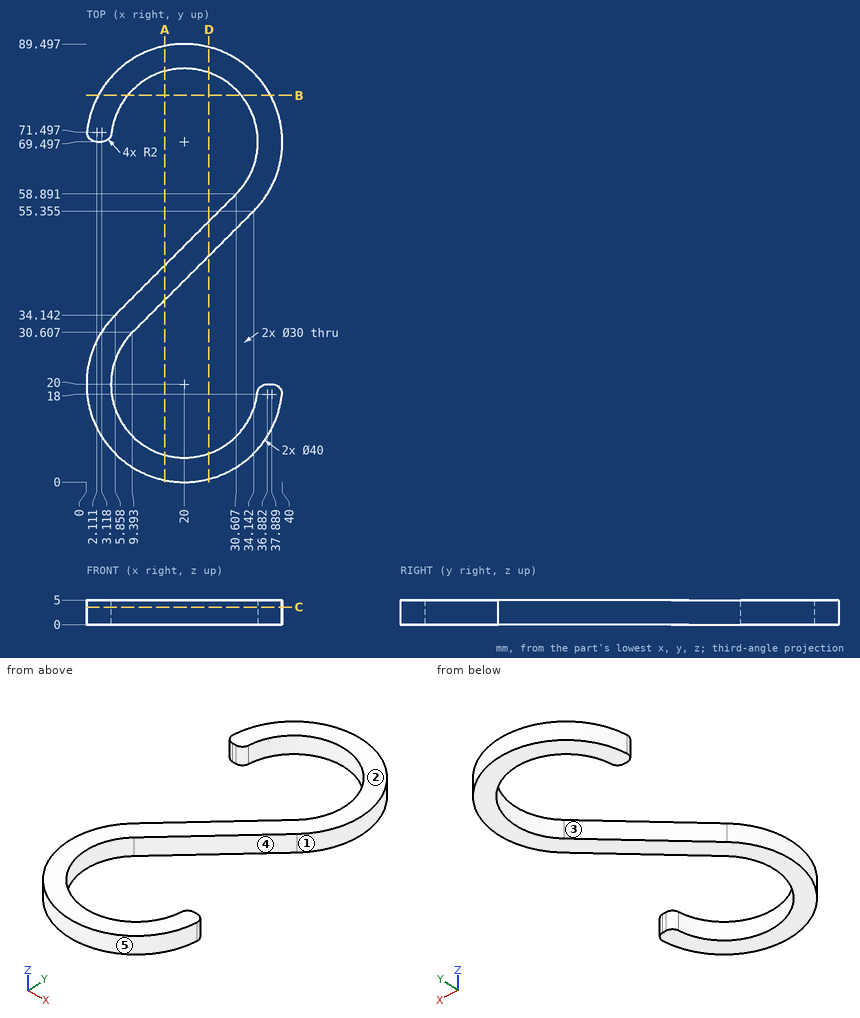
Verification items for this drawing (mm, ordinates from the low corner). A direction names the side the tool comes from. Coordinates: 2 decimals unless noted, no trailing zeros. Loops run counter-clockwise (first coordinate to the right, second up) from the corner with the lowest first, then second, coordinate; pieces in that order, holes last. Notation, with made-up numbers: (-6.75, 4.25) - (0.25, 4.25) arc R29 ccw to (0.25, 29.25) - close; hole circle Ø6 at (36, 73). An arc over 180 degrees is marked (long way). Use one line per item in the form item = value. Start each with the question number.
Item 1: Section check A-A, the plane x = 16. Enter the section's corners in (y, z) (1 decimal).
Item 2: Section check D-D, the plane x = 25. Enter the section's corners in (y, z) (1 decimal).
Item 3: Thickness scan on probe 1 along Y at (x, z) = (26.5, 4.45) (1 decimal); probe 2 along Y at (x, z) = (20, 2.25) (1 decimal); probe 3 along X at (y, z) = (16, 2.4) (1 decimal). Record the ranges inside material, lowest first.
Item 4: Section check C-C, the plane z = 3.6. Enter the section's corners in (x, y) (1 decimal).
Item 5: Gauge pin test, flat ends, axial feed: pin 1 (1.5 mm diameter, centred on y = 19.5, z = 4, fed in from +X); pin 2 (3 mm diameter, centred on y = 34.5, z = 4, fed in from -X); pin 3 (1 mm diameter, centred on y = 70.5, z = 1.5, fed in from +X). Record the tip position at first contact, or that the pin passes through.
Item 6: Mould release check, pull along Y, two halves, no side actions. Record for the marked faces 1 and 2: +Y half, -Y half, draft (parallel to the pull), parting line (faces both ways), or undercut.
Item 7: Tool access check on the marked faces 3, 4 and 5. Record the directions out of +Z, -Z, +X, -X, +Y, -Y that give a thin tool (end or side, any length) a straight path to the whole face; none if there is none.
Item 8: Section check B-B, the plane y = 79. Enter the section's corners in (x, z).
Computed:
q1.outline = (0.4, 0) - (5.5, 0) - (5.5, 5) - (0.4, 5) - close; (37.2, 0) - (44.3, 0) - (44.3, 5) - (37.2, 5) - close; (84, 0) - (89.1, 0) - (89.1, 5) - (84, 5) - close
q2.outline = (0.6, 0) - (5.9, 0) - (5.9, 5) - (0.6, 5) - close; (46.2, 0) - (53.3, 0) - (53.3, 5) - (46.2, 5) - close; (83.6, 0) - (88.9, 0) - (88.9, 5) - (83.6, 5) - close
q3.probe_1 = 1.1 to 6.5, 47.7 to 54.8, 83 to 88.4
q3.probe_2 = 0 to 5, 41.2 to 48.3, 84.5 to 89.5
q3.probe_3 = 0.4 to 5.5, 34.5 to 39.6
q4.outline = (0.1, 71.7) arc R2 ccw to (2.1, 69.5) - (3.1, 69.5) arc R2 ccw to (5.1, 71.3) arc R15 cw (long way) to (30.6, 58.9) - (5.9, 34.1) arc R20 ccw (long way) to (39.9, 17.8) arc R2 ccw to (37.9, 20) - (36.9, 20) arc R2 ccw to (34.9, 18.2) arc R15 cw (long way) to (9.4, 30.6) - (34.1, 55.4) arc R20 ccw (long way) to start
q5.pin_1 = 39.74
q5.pin_2 = 4.8
q5.pin_3 = 39.99
q6.face_1 = undercut
q6.face_2 = draft
q7.face_3 = +Z, -Z, -X
q7.face_4 = +Z, -Z, +X
q7.face_5 = +Z, -Z
q8.outline = (2.4, 0) - (8.39, 0) - (8.39, 5) - (2.4, 5) - close; (31.61, 0) - (37.6, 0) - (37.6, 5) - (31.61, 5) - close
